```python
from build123d import *

# Parameters (mm, degrees)
ESBO_O2_W                = 120
ESBO_O2_H                = 50
RESSALTO_EXTRUS_O1_DEPTH = 20
FILETE1_R                = 6
ESBO_O3_W                = 40
ESBO_O3_H                = 20
CORTE_EXTRUS_O1_DEPTH    = 132.52946438
FILETE2_R                = 6


with BuildPart() as part:
    # Esboço2 → Ressalto-extrusão1 (new body)
    with BuildSketch(Plane(origin=(0, 0, 0), x_dir=(1, 0, 0), z_dir=(0, 1, 0))):
        with Locations((60, 25)):
            Rectangle(ESBO_O2_W, ESBO_O2_H)
    extrude(amount=RESSALTO_EXTRUS_O1_DEPTH)

    # Filete1
    filete1_edges = [part.edges().sort_by_distance(p)[0] for p in [
        (120, 20, -25),
        (60, 20, -50),
        (0, 20, -25),
        (60, 0, -50),
        (120, 0, -25),
        (60, 0, 0),
        (0, 0, -25),
        (60, 20, 0),
    ]]
    fillet(filete1_edges, radius=FILETE1_R)

    # Esboço3 → Corte-extrusão1 (cut, through all)
    with BuildSketch(Plane(origin=(0, 20, 0), x_dir=(1, 0, 0), z_dir=(0, 1, 0))):
        with Locations((79, 25)):
            Rectangle(ESBO_O3_W, ESBO_O3_H)
    extrude(amount=-CORTE_EXTRUS_O1_DEPTH, mode=Mode.SUBTRACT)

    # Filete2
    filete2_edges = [part.edges().sort_by_distance(p)[0] for p in [
        (59, 10, -15),
        (59, 10, -35),
        (99, 10, -35),
        (99, 10, -15),
    ]]
    fillet(filete2_edges, radius=FILETE2_R)


solid = part.part
```
The listing builds one solid part. Answer for the finished solid, in the listing's coordinates (mm). A direction names the side the tool comes from. Round coordinates to 2 decimals unless told otherwise and drop trailing zeros. Loops run counter-clockwise (first coordinate to the right, second up) from the corner with the lowest first, then second, coordinate; pieces in that order, holes last.
Q1. Find the intervals of material crossed by line 1 (Z direction, x = 77, y = 5.75); line 2 (X direction, y = 13.25, z = -19); line 3 (X direction, y = 12.25, z = -33), in increasing order.
Q2. Section D-D, the plane x = 39.5 is taken. Determine the outline of the cut face in (y, z).
Q3. Section B-B, the plane y = 8 is taken. Determine the outline of the cut face in (x, z).
Q4. Section A-A, the plane z = -25 is taken. Determine the outline of the cut face in (x, y).
Q5. For a pull along Z with two mould halves and no side action, classify faces 3 (the face through (59, 10, -25)), 4 (the face through (60.84, 18.196, -1.711)), 5 (the face through (97.196, 9.86, -16.711)), 6 (the face through (1.711, 1.804, -25.35)) as released by +Z, released by -Z, zero draft, split by the parting line, or undercut.
Q6. Which of the six approach directions +Z, -Z, +X, -X, +Y, -Y give full straight-line access (tool end or side, diameter ignored) to faces 1 (the face through (1.711, 18.196, -25.35)), 2 (the face through (79, 10, -15))?
Q7. Section C-C, the plane x = 91 is taken. Determine the outline of the cut face in (y, z), then the cut area to 3 significant figures.
Completed:
1. line 1: z = -49.99 to -35, -15 to -0.01
1. line 2: x = 0 to 59.34, 98.66 to 120
1. line 3: x = 0 to 60.53, 97.47 to 120
2. outline: (0, -44) arc R6 ccw to (6, -50) - (14, -50) arc R6 ccw to (20, -44) - (20, -6) arc R6 ccw to (14, 0) - (6, 0) arc R6 ccw to (0, -6) - close
3. outline: (0, -50) - (120, -50) - (120, 0) - (0, 0) - close; hole (59, -29) arc R6 ccw to (65, -35) - (93, -35) arc R6 ccw to (99, -29) - (99, -21) arc R6 ccw to (93, -15) - (65, -15) arc R6 ccw to (59, -21) - close
4. outline: (0, 6) arc R6 ccw to (6, 0) - (59, 0) - (59, 20) - (6, 20) arc R6 ccw to (0, 14) - close; (99, 0) - (114, 0) arc R6 ccw to (120, 6) - (120, 14) arc R6 ccw to (114, 20) - (99, 20) - close
5. face 3: undercut
5. face 4: released by +Z
5. face 5: undercut
5. face 6: zero draft
6. face 1: +Z, -Z, -X, +Y
6. face 2: +Y, -Y
7. outline: (0, -44) arc R6 ccw to (6, -50) - (14, -50) arc R6 ccw to (20, -44) - (20, -35) - (0, -35) - close; (0, -15) - (20, -15) - (20, -6) arc R6 ccw to (14, 0) - (6, 0) arc R6 ccw to (0, -6) - close
7. area: 569 mm2
